Autodesk Fusion 360 part; units mm, degrees
sketch "Sketch1" plane through (0, 0, 0) normal (1, 0, 0) x (0, 1, 0)
  line L0 (0, 0) -> (250, 0)
  line L1 (250, 0) -> (250, 150)
  line L2 (250, 150) -> (0, 150)
  line L3 (0, 150) -> (0, 0)
  circle A0 centre (0, 75) radius 75
  dimension "d1" = 250
  dimension "d2" = 150
sketch "Sketch2" plane through (0, 0, 0) normal (1, 0, 0) x (0, 1, 0)
extrude "Extrude1" add sketch "Sketch1" along normal blind 150
sketch "Sketch3" plane through (0, 0, 0) normal (-1, 0, 0) x (0, -1, 0)
  line L0 (0, 150) -> (-250, 150)
  line L1 (-250, 150) -> (-250, 0)
  line L2 (-250, 0) -> (0, 0)
  arc A0 (0, 0) -> (0, 150) centre (0, 75) ccw
  line L3 (0, 150) -> (0, 0)
  circle A1 centre (0, 75) radius 37.5
  dimension "d5" = 75
extrude "Extrude2" cut sketch "Sketch3" against normal blind 150 contours L3 A1 | L3 A1
sketch "Sketch4" plane through (150, 0, 0) normal (1, 0, 0) x (0, 1, 0)
  circle A0 centre (0, 75) radius 37.5
  line L0 (250, 150) -> (0, 150)
  arc A1 (0, 150) -> (0, 0) centre (0, 75) ccw
  line L1 (0, 0) -> (250, 0)
  line L2 (250, 0) -> (250, 150)
  line L3 (250, 150) -> (250, 0) construction
  line L4 (250, 75) -> (90, 75) construction
  line L5 (90, 75) -> (90, 100)
  line L6 (90, 75) -> (90, 50)
  line L7 (90, 100) -> (250, 100)
  line L8 (250, 50) -> (90, 50)
  dimension "d8" = 25
  dimension "d9" = 25
extrude "Extrude3" cut sketch "Sketch4" against normal blind 150 contours L2 L5 L6 L7 L8
sketch "Sketch5" plane through (0, 0, 0) normal (0, 0, -1) x (1, 0, 0)
  line L0 (0, 0) -> (0, -250)
  line L1 (0, -250) -> (150, -250)
  line L2 (150, -250) -> (150, 0)
  line L3 (150, 0) -> (0, 0)
  line L4 (0, -250) -> (150, -250) construction
  circle A0 centre (75, -250) radius 75
  dimension "d12" = 150
extrude "Extrude4" add sketch "Sketch5" against normal blind 50 contours L1 A0 picked at (76.8683, -274.9301)
sketch "Sketch6" plane through (0, 0, 0) normal (1, 0, 0) x (0, 1, 0)
  line L0 (220, 110) -> (210, 110)
  line L1 (250, 150) -> (250, 20) construction
sketch "Sketch7" plane through (0, 0, 150) normal (0, 0, 1) x (-1, 0, 0)
  line L0 (0, -250) -> (0, 0)
  line L1 (0, 0) -> (-150, 0)
  line L2 (-150, 0) -> (-150, -250)
  line L3 (-150, -250) -> (0, -250)
  circle A0 centre (-75, -250) radius 75
  dimension "d15" = 150
extrude "Extrude5" add sketch "Sketch7" against normal blind 50 contours L3 A0 picked at (-76.8683, -274.9301)
sketch "Sketch8" plane through (0, 0, 150) normal (0, 0, 1) x (-1, 0, 0)
  line L0 (0, -250) -> (0, 0)
  line L1 (0, 0) -> (-150, 0)
  line L2 (-150, 0) -> (-150, -250)
  arc A0 (-150, -250) -> (0, -250) centre (-75, -250) ccw
  circle A1 centre (-75.6677, -249.6068) radius 37.5
  dimension "d18" = 75
extrude "Extrude6" cut sketch "Sketch8" against normal blind 50 contours A1
sketch "Sketch9" plane through (0, 0, 0) normal (0, 0, -1) x (1, 0, 0)
  line L0 (0, 0) -> (0, -250)
  arc A0 (0, -250) -> (150, -250) centre (75, -250) ccw
  line L1 (150, -250) -> (150, 0)
  line L2 (150, 0) -> (0, 0)
  circle A1 centre (75, -250) radius 37.5
  line L3 (0, -250) -> (150, -250) construction
  dimension "d21" = 75
extrude "Extrude7" cut sketch "Sketch9" against normal blind 50 contours A1
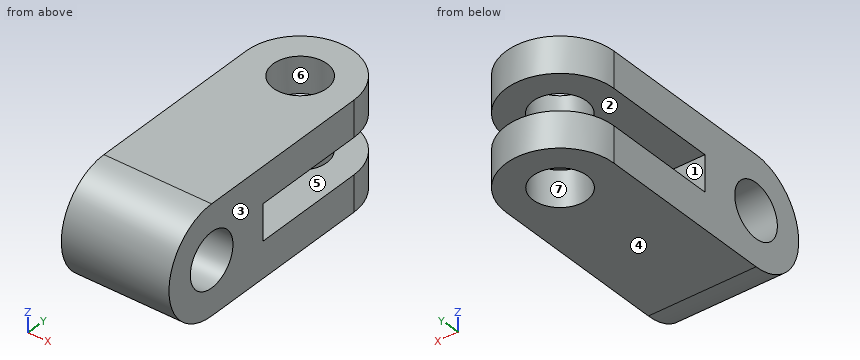
The listing builds one solid part. Answer for the finished solid, in the listing's coordinates (mm). Face numbers are marked on the shaded views. A direction names the side the tool comes from. Coordinates: 2 decimals unless noted, no trailing zeros. Write each loop counter-clockwise with the first axis right and the second up, starting at its lowest first coordinate (ties: lowest second). Pieces come first, ordered by that corner, then holes. Notation, with made-up numbers: (24, 25.25) -> (59, 25.25) arc R15 ccw to (59, 50.25) -> close; hole circle Ø3 at (46, 82). An arc over 180 degrees is marked (long way). Write each question's results on one line, items separated by ' | '. Start each with the question number.
1) A tool of negligible diameter and unlimited length cuts with its end or side. For the marked faces 5, 6 and 7, from which of +Z, -Z, +X, -X, +Y, -Y can it reach the whole face along a straight path? Write none if from no direction.
2) A cutting plane is placed at B-B (x = 100). Determine the outline of the cut face in (y, z), then the cut area to 3 significant figures.
3) A cutting plane is placed at A-A (z = 75). Determine the outline of the cut face in (x, y), then the cut area to 3 significant figures.
4) Straight lines are drawn through the part: probe 1 along Z at (x, y) = (22.5, 291); probe 2 along X at (y, z) = (250, 29); probe 3 along Y at (x, z) = (76, 126). For each, find the intervals that lie inside material, in ascending order.
5) A cutting plane is placed at D-D (z = 104.5). Determine the outline of the cut face in (x, y).
6) A cutting plane is placed at C-C (y = 268). Determine the outline of the cut face in (x, z), then the cut area to 3 significant figures.
7) Flat-ended cylindrical pins translate along their axes: pin 1 Ø15 at (x, z) = (78.5, 64) entering from +Y; pin 2 Ø6 at (x, z) = (70, 38.5) entering from +Y; pin 3 Ø1 at (x, z) = (39.5, 122) entering from +Y. Find the tip coordinate at first contact, or state that the pin passes through.
8) For a pull along Z with two mould halves and no side action, classify the marked faces 1, 2, 3 and 4 as +Z half, -Z half, draft (parallel to the pull), parting line (faces both ways), or undercut.
Values follow:
1) face 5: +X, -X, +Y | face 6: +Z | face 7: -Z
2) outline: (0, 0) -> (222.05, 0) -> (222.05, 50) -> (90, 50) -> (90, 100) -> (221.07, 100) -> (221.07, 150) -> (0, 150) arc R75 ccw to start; (277.95, 0) -> (320.71, 0) -> (320.71, 50) -> (277.95, 50) -> close; (278.14, 100) -> (320.71, 100) -> (320.71, 150) -> (278.14, 150) -> close; hole circle Ø75 at (0, 75) | area: 35,300 mm²
3) outline: (0, -75) -> (150, -75) -> (150, -37.5) -> (0, -37.5) -> close; (0, 37.5) -> (150, 37.5) -> (150, 90) -> (0, 90) -> close | area: 13,500 mm²
4) probe 1: 0 to 50, 100 to 150 | probe 2: 0 to 37.5, 112.5 to 150 | probe 3: -54.99 to 212.11, 287.11 to 324.99
5) outline: (0, -68.95) -> (150, -68.95) -> (150, -23.15) -> (0, -23.15) -> close; (0, 23.15) -> (150, 23.15) -> (150, 250) arc R75 ccw to (0, 250) -> close; hole circle Ø75 at (75.67, 249.61)
6) outline: (2.19, 0) -> (42.1, 0) -> (42.1, 50) -> (2.19, 50) -> close; (2.19, 100) -> (42.99, 100) -> (42.99, 150) -> (2.19, 150) -> close; (107.9, 0) -> (147.81, 0) -> (147.81, 50) -> (107.9, 50) -> close; (108.35, 100) -> (147.81, 100) -> (147.81, 150) -> (108.35, 150) -> close | area: 8,000 mm²
7) pin 1: y = 90 | pin 2: y = 324.97 | pin 3: y = 316.33
8) face 1: undercut | face 2: undercut | face 3: draft | face 4: -Z half
